```python
from build123d import *

# Parameters (mm, degrees)
SKIZZE2_R                        = 15
AUFSATZ_LINEAR_AUSTRAGEN1_DEPTH  = 20
F_10_0_10_DURCHMESSER_BOHRUNG1_D = 10
F_5_0_5_DURCHMESSER_BOHRUNG1_D   = 5


with BuildPart() as part:
    # Skizze2 → Aufsatz-Linear austragen1 (new body)
    with BuildSketch(Plane.XY):
        Circle(SKIZZE2_R)
    extrude(amount=AUFSATZ_LINEAR_AUSTRAGEN1_DEPTH)

    # Ø10.0 (10) Durchmesser Bohrung1 (through all)
    with Locations(Plane.XY.offset(20)):
        with Locations((0, 0)):
            Hole(F_10_0_10_DURCHMESSER_BOHRUNG1_D / 2)

    # Ø5.0 (5) Durchmesser Bohrung1 (through all)
    with Locations(Plane.XY.offset(20)):
        with Locations((-7.5, 7.5), (7.5, -7.5)):
            Hole(F_5_0_5_DURCHMESSER_BOHRUNG1_D / 2)


solid = part.part
```
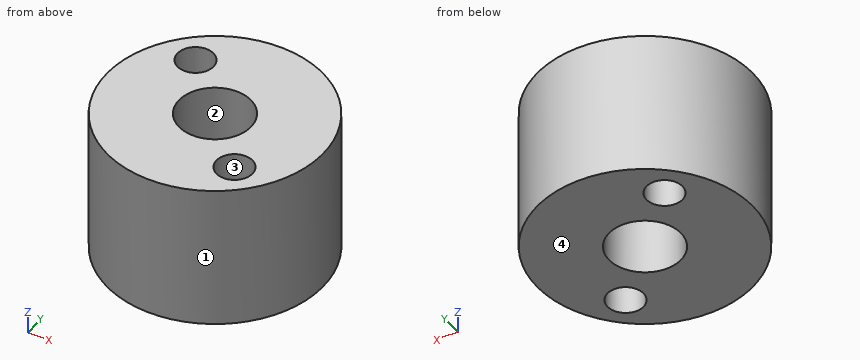
The listing builds one solid part. Answer for the finished solid, in the listing's coordinates (mm). Face numbers are marked on the shaded views. Give positions to 0.01 mm unless a question says otherwise; leave off trailing zeros. Order: outer loops, then holes, each group sorted by start corner. A loop starts at its lowest first (then second) coordinate and runs counter-clockwise, first axis right, second up. Notation, with made-up numbers: (28, 67.25) - (51, 67.25) arc R32 cw to (51, 95.25) - close; hole circle Ø1 at (-34.5, 63.5). An arc over 180 degrees is marked (long way). Answer in a Markdown table with one row per item. Add a question column.
Q1. The part is cut by section D-D (y = 12). Determine the outline of the cut face in (x, z).
Q2. The part is cut by section B-B (x = 6.5). Determine the outline of the cut face in (y, z), then the cut area to 3 significant figures.
Q3. Find the intervals of material crossed by line 1 along Y through (x, z) = (0, 13.5); line 2 along Y through (x, z) = (-2, 8.5); line 3 along X through (y, z) = (9.5, 18), in increasing order. Write a range as [from, to].
Q4. For a pull along Y with two mould halves and no side action, classify the marked faces 1, 2, 3 and 4 as released by +Y, released by -Y, zero draft, split by the parting line, or undercut.
Q5. The part is cut by section A-A (y = 0). Determine the outline of the cut face in (x, z), then the cut area to 3 significant figures.
Q6. The part is cut by section C-C (z = 10). Determine the outline of the cut face in (x, y).
Q7. Given P1, Ø4, axis at x = 5, z = 13, coming from the -Y side; P2, Ø3, axis at x = -7.5, y = 7.5, coming from the +Z side; P3, Ø8, axis at x = -7.5, z = 17, coming from the -Y side; P4, Ø2, axis at y = -8, z = 3.5, coming from the -X side, each flat-ended and moving along its own axis, determine where each tip first touches the part or whether it passes through.
Determined:
| question | item | result |
|---|---|---|
| 1 | outline | (-9, 0) - (9, 0) - (9, 20) - (-9, 20) - close |
| 2 | outline | (-13.52, 0) - (-9.79, 0) - (-9.79, 20) - (-13.52, 20) - close; (-5.21, 0) - (13.52, 0) - (13.52, 20) - (-5.21, 20) - close |
| 2 | area | 449 mm² |
| 3 | line 1 | y = [-15, -5], [5, 15] |
| 3 | line 2 | y = [-14.87, -4.58], [4.58, 14.87] |
| 3 | line 3 | x = [-11.61, -9], [-6, 11.61] |
| 4 | face 1 | split by the parting line |
| 4 | face 2 | undercut |
| 4 | face 3 | undercut |
| 4 | face 4 | zero draft |
| 5 | outline | (-15, 0) - (-5, 0) - (-5, 20) - (-15, 20) - close; (5, 0) - (15, 0) - (15, 20) - (5, 20) - close |
| 5 | area | 400 mm² |
| 6 | outline | circle Ø30 at (0, 0); hole circle Ø5 at (-7.5, 7.5); hole circle Ø10 at (0, 0); hole circle Ø5 at (7.5, -7.5) |
| 7 | P1 | stops at y = -14.7 |
| 7 | P2 | passes through |
| 7 | P3 | stops at y = -14.59 |
| 7 | P4 | stops at x = -13.27 |
